Verification items for the finished model (mm, model axes). A direction names the side the tool comes from. Round coordinates to 2 decimals unless told otherwise and drop trailing zeros. Order: outer loops, then holes, each group sorted by start corner. A loop starts at its lowest first (then second) coordinate and runs counter-clockwise, first axis right, second up.
```python
from build123d import *

# Parameters (mm, degrees)
BOSS_EXTRUDE1_DEPTH = 60
SKETCH4_W           = 10
SKETCH4_H           = 1.497685239
BOSS_EXTRUDE2_DEPTH = 60
SKETCH6_W           = 10
SKETCH6_H           = 18.014625213
BOSS_EXTRUDE3_DEPTH = 5
CUT_EXTRUDE1_DEPTH  = 10
SKETCH8_W           = 18.010643645
SKETCH8_H           = 57.5
BOSS_EXTRUDE4_DEPTH = 1


with BuildPart() as part:
    # Sketch2 → Boss-Extrude1 (new body)
    with BuildSketch(Plane(origin=(0, 0, 0), x_dir=(1, 0, 0), z_dir=(0, 1, 0))):
        Polygon((-22, -22), (-22, -12), (-12, -22), align=None)
    extrude(amount=BOSS_EXTRUDE1_DEPTH)



with BuildPart() as body_2:
    # Sketch4 → Boss-Extrude2 (new body)
    with BuildSketch(Plane.XZ):
        with Locations((-17, 40.763467832)):
            Rectangle(SKETCH4_W, SKETCH4_H)
    extrude(amount=-BOSS_EXTRUDE2_DEPTH)


with BuildPart() as part_1:
    add(part.part)

    add(body_2.part)  # Boss-Extrude3 merges body 2
    # Sketch6 → Boss-Extrude3 (add)
    with BuildSketch(Plane(origin=(0, 0, 0), x_dir=(-1, 0, 0), z_dir=(0, -1, 0))):
        with Locations((17, -31.007312607)):
            Rectangle(SKETCH6_W, SKETCH6_H)
    boss_extrude3 = extrude(amount=-BOSS_EXTRUDE3_DEPTH)

    # Mirror1: Boss-Extrude3 across plane
    add(boss_extrude3.mirror(Plane.ZX.offset(30)))

    # Sketch7 → Cut-Extrude1 (cut)
    with BuildSketch(Plane(origin=(-12, 0, 0), x_dir=(0, 0, -1), z_dir=(1, 0, 0))):
        Polygon((-40.014625213, 55), (-22, 55), (-22, 57.5), (-22, 58.75), (-40.014625213, 58.75), (-40.014625213, 57.5), align=None)
        Polygon((-22, 2.5), (-22, 5), (-40.014625213, 5), (-40.010643645, 2.5), (-40.010643645, 1.25), (-22, 1.25), align=None)
    extrude(amount=-CUT_EXTRUDE1_DEPTH, mode=Mode.SUBTRACT)

    # Sketch8 → Boss-Extrude4 (add)
    with BuildSketch(Plane.ZY.offset(22)):
        with Locations((31.005321823, 30)):
            Rectangle(SKETCH8_W, SKETCH8_H)
    extrude(amount=-BOSS_EXTRUDE4_DEPTH)


solid = part_1.part
```
1) Tool access check on faces 1 (the flat face through (-21, 30, 31)), 2 (the flat face through (-17, 0, 30)). Record the directions out of +Z, -Z, +X, -X, +Y, -Y that give a thin tool (end or side, any length) a straight path to the whole face; none if there is none.
2) Sectioned sample at A-A on y = 39. Record the cut outline in (x, z).
3) Draft check along Z on faces 3 (the flat face through (-17, 30, 41.512)), 4 (the flat face through (-12, 39, 40.5)), 5 (the flat face through (-16, 30, 22)). Enter one of: released by +Z, released by -Z, zero draft, split by the parting line, or undercut.
4) Go/stop test with flat-tipped pins: pin 1 Ø1 at (x, y) = (-16.5, 2) entering from -Z; pin 2 Ø2 at (x, y) = (-16.5, 52) entering from -Z; pin 3 Ø2 at (x, y) = (-13.5, 41) entering from -Z. Record where each tip stops, or that it passes through.
5) Sectioned sample at D-D on x = -18.5. Record the cut outline in (y, z), then the cut area to 3 significant figures.
6) Sectioned sample at B-B on x = -15.25. Record the cut outline in (y, z), then the cut area to 3 significant figures.
7) Sectioned sample at C-C on z = 36.5. Record the cut outline in (x, y), then the cut area to 3 significant figures.
8) Scan lines: probe 1 along Y at (x, z) = (-19.5, 22.5); probe 2 along X at (y, z) = (27.5, 34.5); probe 3 along Z at (x, y) = (-13.5, 24). Record each from-to range of solid material in increasing order.
Returned:
1. face 1: +X
1. face 2: +Z, -Z, +X, -X, -Y
2. outline: (-22, 12) - (-12, 22) - (-21, 22) - (-21, 40.01) - (-22, 40.01) - close; (-22, 40.01) - (-12, 40.01) - (-12, 41.51) - (-22, 41.51) - close
3. face 3: released by +Z
3. face 4: zero draft
3. face 5: undercut
4. pin 1: stops at z = 17
4. pin 2: stops at z = 16.5
4. pin 3: stops at z = 19.5
5. outline: (0, 15.5) - (60, 15.5) - (60, 41.51) - (0, 41.51) - close; hole (1.25, 22) - (58.75, 22) - (58.75, 40.01) - (5, 40.01) - (2.5, 40.01) - (1.25, 40.01) - close
5. area: 525 mm2
6. outline: (0, 18.75) - (60, 18.75) - (60, 41.51) - (0, 41.51) - close; hole (1.25, 22) - (58.75, 22) - (58.75, 40.01) - (5, 40.01) - (2.5, 40.01) - (1.25, 40.01) - close
6. area: 330 mm2
7. outline: (-22, 0) - (-12, 0) - (-12, 1.25) - (-21, 1.25) - (-21, 58.75) - (-12, 58.75) - (-12, 60) - (-22, 60) - close
7. area: 82.5 mm2
8. probe 1: y = 0 to 1.25, 58.75 to 60
8. probe 2: x = -22 to -21
8. probe 3: z = 20.5 to 22, 40.01 to 41.51
